Verification items for the finished model (mm, model axes). Face numbers are marked on the shaded views. A direction names the side the tool comes from. Coordinates: 2 decimals unless noted, no trailing zeros. Loops run counter-clockwise (first coordinate to the right, second up) from the corner with the lowest first, then second, coordinate; pieces in that order, holes last. Notation, with made-up numbers: (-37.75, 83.25) -> (21.25, 83.25) arc R28 cw to (21.25, 122.25) -> close; hole circle Ø5 at (38.25, 41). An arc over 180 degrees is marked (long way). Use CSV: the item, a comma, the result in double quotes. Start each with the question number.
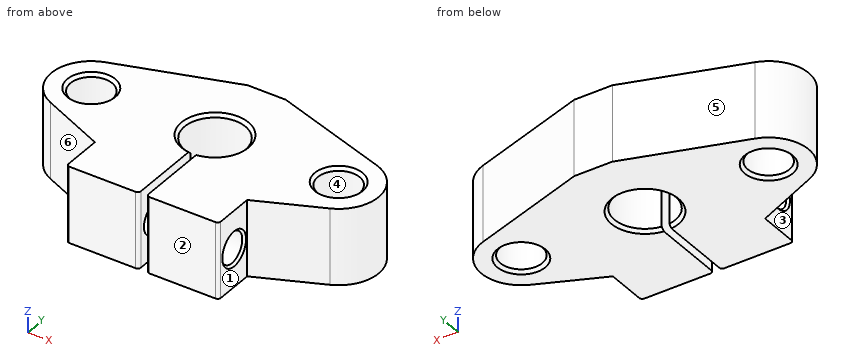
```python
from build123d import *

# Parameters (mm, degrees)
SKETCH_R        = 4
SKETCH_R_2      = 2.75
PAD_DEPTH       = 5
SKETCH001_W     = 1
SKETCH001_H     = 12
POCKET_DEPTH    = 10.001
CHAMFER_SIZE    = 0.4
FILLET_R        = 0.4
SKETCH002_R     = 2
POCKET001_DEPTH = 31.501
CHAMFER001_SIZE = 0.3


with BuildPart() as part:
    # Sketch → Pad (new body, symmetric)
    with BuildSketch(Plane.XY):
        with BuildLine():
            Line((-2.5, 10), (2.5, 10))
            Line((17.875915, 4.991883), (2.5, 10))
            ThreePointArc((18.371237, -4.80238), (21.493299, 0.265167), (17.875915, 4.991883))
            Line((18.371237, -4.80238), (10, -8.5))
            Line((10, -14), (10, -8.5))
            Line((-10, -14), (10, -14))
            Line((-10, -14), (-10, -8.5))
            Line((-10, -8.5), (-18.371237, -4.80238))
            ThreePointArc((-17.875915, 4.991883), (-21.493299, 0.265167), (-18.371237, -4.80238))
            Line((-17.875915, 4.991883), (-2.5, 10))
        make_face()
        Circle(SKETCH_R, mode=Mode.SUBTRACT)
        with Locations((16.25, 0)):
            Circle(SKETCH_R_2, mode=Mode.SUBTRACT)
        with Locations((-16.25, 0)):
            Circle(SKETCH_R_2, mode=Mode.SUBTRACT)
    extrude(amount=PAD_DEPTH, both=True)

    # Sketch001 (on Face15 of Pad) → Pocket (cut, through all)
    with BuildSketch(Plane.XY.offset(5)):
        with Locations((0, -9)):
            Rectangle(SKETCH001_W, SKETCH001_H)
    extrude(amount=-POCKET_DEPTH, mode=Mode.SUBTRACT)

    # Chamfer
    chamfer_edges = [part.edges().sort_by_distance(p)[0] for p in [
        (-19, 0, 5),
        (13.5, 0, 5),
        (-19, 0, -5),
        (13.5, 0, -5),
        (-2.645751, 3, -5),
        (-2.645751, 3, 5),
    ]]
    chamfer(chamfer_edges, length=CHAMFER_SIZE)

    # Fillet
    fillet_edges = [part.edges().sort_by_distance(p)[0] for p in [
        (10, -14, 0),
        (0.5, -14, 0),
        (-0.5, -14, 0),
        (-10, -14, 0),
    ]]
    fillet(fillet_edges, radius=FILLET_R)

    # Sketch002 (on Face16 of Fillet) → Pocket001 (cut, through all)
    with BuildSketch(Plane.YZ.offset(10)):
        with Locations((-11, 0)):
            Circle(SKETCH002_R)
    extrude(amount=-POCKET001_DEPTH, mode=Mode.SUBTRACT)

    # Chamfer001
    chamfer001_edges = [part.edges().sort_by_distance(p)[0] for p in [
        (10, -13, 0),
        (-10, -13, 0),
    ]]
    chamfer(chamfer001_edges, length=CHAMFER001_SIZE)


solid = part.part
```
1. Release check for a two-part mould opening along Y. For the marked faces 4, 5 and 6 record: released by +Y, released by -Y, zero draft, split by the parting line, or undercut.
2. Cross-section at C-C, the plane x = -16.25. Record the boundary of the cut face in (y, z), plus the area to 3 significant figures.
3. Scan lines: line 1 (Y direction, x = 1.5, z = 1.25); line 2 (X direction, y = 2.5, z = 4); line 3 (Y direction, x = 0, z = 1.25). Record each from-to range of solid material in increasing order.
4. Set-up check for the marked faces 1, 2 and 3: record each of +Z, -Z, +X, -X, +Y, -Y from which the full face is reachable in a straight line by a thin tool's end or side.
5. Depth check by flat-ended pin: pin 1 (5 mm diameter, centred on y = 4.5, z = 0.5, fed in from -X); pin 2 (12 mm diameter, centred on x = 16, y = 1, fed in from +Z); pin 3 (4 mm diameter, centred on y = -12, z = 2, fed in from +X); pin 4 (3 mm diameter, centred on x = 8, z = -1, fed in from +Y). Enter the tip coordinate at first touch or a pass-through.
6. Cross-section at A-A, the plane z = 0. State how many separate pieces and enclosed holes the cut face has, plus the area to 3 significant figures.
7. Cross-section at D-D, the plane y = -11. Record the boundary of the cut face in (x, z), plus the area to 3 significant figures.
8. Cross-section at B-B, the plane y = 0. Record the boundary of the cut face in (x, z), plus the area to 3 significant figures.
Solution:
1,face 4,"undercut"
1,face 5,"released by +Y"
1,face 6,"released by -Y"
2,outline,"(-5.74, -5) -> (-3.15, -5) -> (-2.75, -4.6) -> (-2.75, 4.6) -> (-3.15, 5) -> (-5.74, 5) -> close; (2.75, -4.6) -> (3.15, -5) -> (5.52, -5) -> (5.52, 5) -> (3.15, 5) -> (2.75, 4.6) -> close"
2,area,"57.3 mm2"
3,line 1,"y = -14 to -12.56, -9.44 to -3.71, 3.71 to 10"
3,line 2,"x = -20.87 to -17.4, -15.1 to -3.12, 3.12 to 15.1, 17.4 to 20.87"
3,line 3,"y = 4 to 10"
4,face 1,"+Z, -Z, +X, -Y"
4,face 2,"+Z, -Z, +X, -X, -Y"
4,face 3,"+Z, -Z, -X, -Y"
5,pin 1,"stops at x = -21.1"
5,pin 2,"stops at z = 5"
5,pin 3,"stops at x = 10"
5,pin 4,"stops at y = 8.7"
6,separate pieces,"3"
6,enclosed holes,"2"
6,area,"536 mm2"
7,outline,"(-10, -5) -> (-0.5, -5) -> (-0.5, -2) -> (-9.7, -2) -> (-10, -2.3) -> close; (-10, 2.3) -> (-9.7, 2) -> (-0.5, 2) -> (-0.5, 5) -> (-10, 5) -> close; (0.5, -5) -> (10, -5) -> (10, -2.3) -> (9.7, -2) -> (0.5, -2) -> close; (0.5, 2) -> (9.7, 2) -> (10, 2.3) -> (10, 5) -> (0.5, 5) -> close"
7,area,"114 mm2"
8,outline,"(-21.5, -5) -> (-19.4, -5) -> (-19, -4.6) -> (-19, 4.6) -> (-19.4, 5) -> (-21.5, 5) -> close; (-13.5, -4.6) -> (-13.1, -5) -> (-4.4, -5) -> (-4, -4.6) -> (-4, 4.6) -> (-4.4, 5) -> (-13.1, 5) -> (-13.5, 4.6) -> close; (4, -4.6) -> (4.4, -5) -> (13.1, -5) -> (13.5, -4.6) -> (13.5, 4.6) -> (13.1, 5) -> (4.4, 5) -> (4, 4.6) -> close; (19, -4.6) -> (19.4, -5) -> (21.5, -5) -> (21.5, 5) -> (19.4, 5) -> (19, 4.6) -> close"
8,area,"239 mm2"
